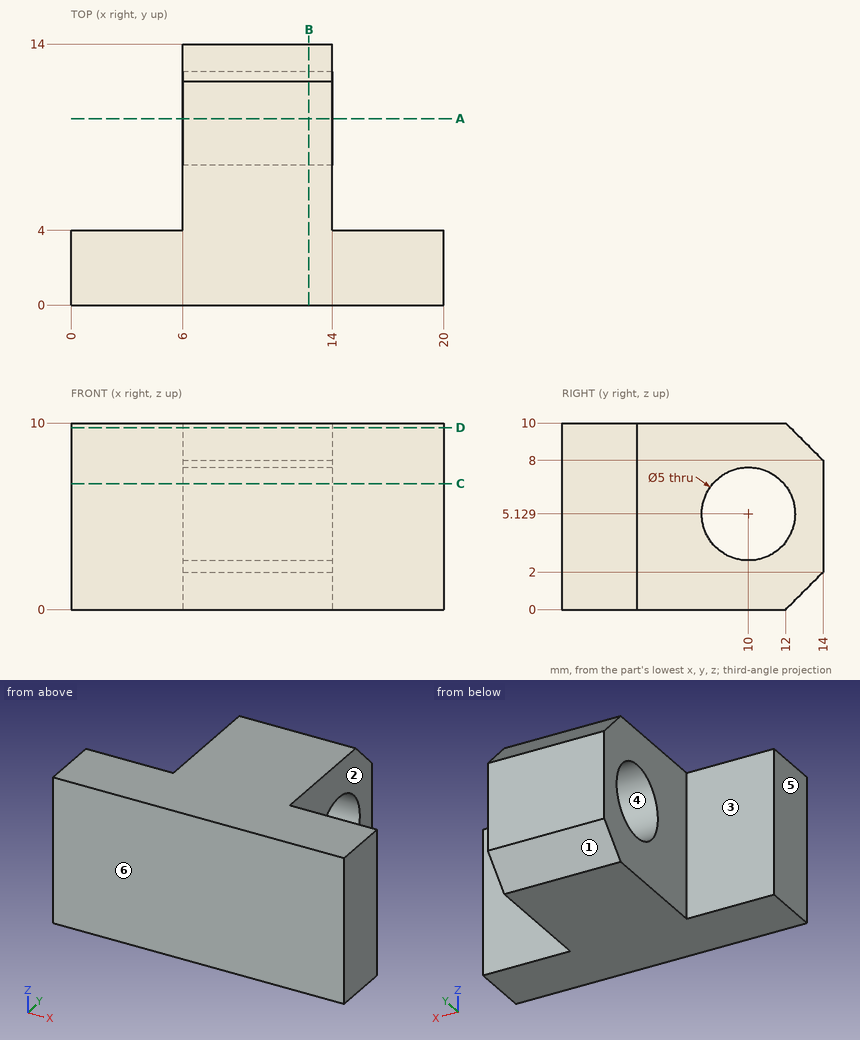
Drawing for the job (mm, zero at the part's lowest x, y, z). A direction names the side the tool comes from. Coordinates: 2 decimals unless noted, no trailing zeros. Order: outer loops, then holes, each group sorted by start corner. A loop starts at its lowest first (then second) coordinate and runs counter-clockwise, first axis right, second up. Notation, with made-up numbers: (-10.75, 62) - (46.25, 62) arc R30 ccw to (46.25, 90) - close; hole circle Ø3 at (80, 87). An arc over 180 degrees is marked (long way). Use a Markdown table: item, result. Add a question column.
(1) Drill centre lines: line 1 along X through (y, z) = (4.25, 8); line 2 along Y through (x, z) = (5.75, 8.5); line 3 along Y through (x, z) = (13.75, 4.5). Where is each one in solid material? Low to high. Write a range as [from, to].
(2) Saw through at B-B (x = 12.75). Give the cut face in (y, z), then the cut area to 3 significant figures.
(3) Pull direction Y, two halves, no side cores. Call the marked faces 4, 5 and 6: +Y half, -Y half, draft (parallel to the pull), parting line (faces both ways), or undercut.
(4) Flat gauge pins, fed straight in: pin 1 (3 mm diameter, centred on y = 9, z = 8, fed in from +X); pin 2 (5 mm diameter, centred on x = 1.5, z = 3, fed in from +Y). Where does each tip first touch, or does it go through?
(5) Saw through at D-D (z = 9.75). Give the cut face in (x, y).
(6) Which spindle directions (+Z, -Z, +X, -X, +Y, -Y) get a long thin tool onto all of the face, cutting with end or side? Do the marked faces 1, 2 and 3. Say none if no direction does.
(7) Saw through at A-A (y = 10). Give the cut face in (x, z).
(8) Saw through at C-C (z = 6.75). Give the cut face in (x, y).
Solved:
| question | item | result |
|---|---|---|
| 1 | line 1 | x = [6, 14] |
| 1 | line 2 | y = [0, 4] |
| 1 | line 3 | y = [0, 7.58], [12.42, 14] |
| 2 | outline | (0, 0) - (12, 0) - (14, 2) - (14, 8) - (12, 10) - (0, 10) - close; hole circle Ø5 at (10, 5.13) |
| 2 | area | 116 mm² |
| 3 | face 4 | undercut |
| 3 | face 5 | draft |
| 3 | face 6 | -Y half |
| 4 | pin 1 | stops at x = 14 |
| 4 | pin 2 | stops at y = 4 |
| 5 | outline | (0, 0) - (20, 0) - (20, 4) - (14, 4) - (14, 12.25) - (6, 12.25) - (6, 4) - (0, 4) - close |
| 6 | face 1 | -Z, +X, -X, +Y |
| 6 | face 2 | +Z, -Z, +X, +Y |
| 6 | face 3 | +Z, -Z, -X, +Y |
| 7 | outline | (6, 0) - (14, 0) - (14, 2.63) - (6, 2.63) - close; (6, 7.63) - (14, 7.63) - (14, 10) - (6, 10) - close |
| 8 | outline | (0, 0) - (20, 0) - (20, 4) - (14, 4) - (14, 8.1) - (6, 8.1) - (6, 4) - (0, 4) - close; (6, 11.9) - (14, 11.9) - (14, 14) - (6, 14) - close |
